Verification items for the finished model (mm, model axes). Face numbers are marked on the shaded views. Coordinates: 2 decimals unless noted, no trailing zeros. Order: outer loops, then holes, each group sorted by start corner. A loop starts at its lowest first (then second) coordinate and runs counter-clockwise, first axis right, second up. Notation, with made-up numbers: M 85.25,46.5 L 94.25,46.5 A17 cw 94.25,54.5 Z; hole C 65.5,55.5 d10. An arc over 180 degrees is marked long. Return JSON: item names as keys, results as strings. Group by question number.
Q1. Mould release check, pull along X, two halves, no side actions. Record for the marked faces 1, 2, 3 and 4: pulls with the +X half, pulls with the -X half, needs draft (parallel to the pull), parting line crosses it, or undercut.
Q2. Go/stop test with flat-tipped pins: pin 1 Ø4 at (x, z) = (43.5, 1.5) entering from +Y; pin 2 Ø1 at (x, z) = (21, 2) entering from -Y; pin 3 Ø8 at (x, y) = (33.5, -4) entering from +Z. Record where each tip stops, or that it passes through.
Q3. Section check C-C, the plane x = 45. Enter the section's corners in (y, z).
Q4. Thickness scan on probe 1 along X at (y, z) = (6, -27); probe 2 along X at (y, z) = (20.5, 14.5); probe 3 along X at (y, z) = (18, -12.5). Record the ranges inside material, lowest first.
Q5. Section check D-D, the plane x = 36. Enter the section's corners in (y, z).
Q6. Section check A-A, the plane y = 0. Enter the section's corners in (x, z), then the cut area to 3 significant figures.
from build123d import *

# Parameters (mm, degrees)
SKETCH1_R        = 30
BIGLIP_DEPTH     = 6
SKETCH2_R        = 27
INNERTUBE_DEPTH  = 33
SKETCH3_R        = 21.5
CONNECTION_DEPTH = 4
SKETCH4_R        = 24.5
SMALLLIP_DEPTH   = 6
CHAMFER1_SIZE    = 3.119205001
CHAMFER1_SIZE_2  = 0.55


with BuildPart() as part:
    # Sketch1 → bigLip (new body)
    with BuildSketch(Plane(origin=(0, 0, 0), x_dir=(0, 0, -1), z_dir=(1, 0, 0))):
        Circle(SKETCH1_R)
    extrude(amount=BIGLIP_DEPTH)

    # Sketch2 → innerTube (add)
    with BuildSketch(Plane(origin=(6, 0, 0), x_dir=(0, 0, -1), z_dir=(1, 0, 0))):
        Circle(SKETCH2_R)
    extrude(amount=INNERTUBE_DEPTH)

    # Sketch3 → connection (add)
    with BuildSketch(Plane(origin=(39, 0, 0), x_dir=(0, 0, -1), z_dir=(1, 0, 0))):
        Circle(SKETCH3_R)
    extrude(amount=CONNECTION_DEPTH)

    # Sketch4 → smallLip (add)
    with BuildSketch(Plane(origin=(43, 0, 0), x_dir=(0, 0, -1), z_dir=(1, 0, 0))):
        Circle(SKETCH4_R)
    extrude(amount=SMALLLIP_DEPTH)

    # Chamfer1
    # the kernel refuses this chamfer: 3.119205001, 0.55 mm, written as the material it adds along each edge
    with BuildSketch(Plane(origin=(43, 0, 0), x_dir=(0, 0, -1), z_dir=(0, -1, 0))) as chamfer1_piece_1_section:
        Polygon((21.5 + CHAMFER1_SIZE, 0), (21.5, -CHAMFER1_SIZE_2), (21.5, 0), align=None)
    chamfer1_piece_1 = revolve(axis=Axis((43, 0, 0), (1, 0, 0)), mode=Mode.PRIVATE)
    chamfer1_piece_1 = chamfer1_piece_1 & Plane(origin=(42.756656471, 0, 0), x_dir=(0, 0, -1), z_dir=(-1, 0, 0)) * Cylinder(24.5, 99, mode=Mode.PRIVATE)
    add(chamfer1_piece_1)


solid = part.part
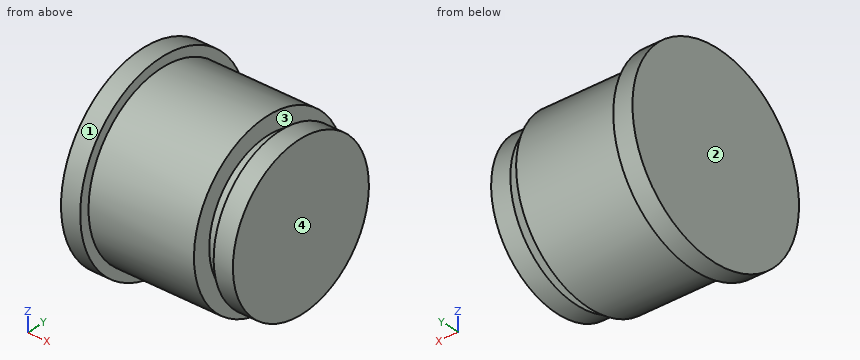
Numbers:
{
 "1": {"face 1": "needs draft", "face 2": "pulls with the -X half", "face 3": "undercut", "face 4": "pulls with the +X half"},
 "2": {"pin 1": "stops at y = 24.5", "pin 2": "stops at y = -26.96", "pin 3": "stops at z = 27"},
 "3": {"outline": "C 0,0 d49"},
 "4": {"probe 1": "x = 0 to 6", "probe 2": "x = 0 to 39", "probe 3": "x = 0 to 39, 42.52 to 49"},
 "5": {"outline": "C 0,0 d54"},
 "6": {"outline": "M 0,-30 L 6,-30 L 6,-27 L 39,-27 L 39,-21.5 L 42.45,-21.5 L 42.98,-24.5 L 49,-24.5 L 49,24.5 L 42.98,24.5 L 42.45,21.5 L 39,21.5 L 39,27 L 6,27 L 6,30 L 0,30 Z", "area": "2,610 mm2"}
}
